Build history of the part. All positions in model axes, mm. A direction names the side the tool comes from. Round coordinates to 2 decimals unless told otherwise and drop trailing zeros. Write each loop counter-clockwise with the first axis right and the second up, starting at its lowest first coordinate (ties: lowest second). Pieces come first, ordered by that corner, then holes. Notation, with made-up numbers: M -38.75,66.25 L -1.75,66.25 A7 ccw -1.75,79.25 Z; hole C 47,-31.5 d10. An arc over 180 degrees is marked long. Write item = value, one per line. Start each with the question number.
Q1. Drop flat-ended pins along their axis: P1, Ø2.5, axis at x = -21.5, y = 1.5, coming from the +Z side; P2, Ø3.5, axis at y = 50.5, z = -25.11, coming from the -X side; P3, Ø5.5, axis at y = 1.5, z = 38.5, coming from the -X side; P4, Ø5.5, axis at x = -17.32, z = 10, coming from the -Y side. Give the stop position or say it passes through.
Q2. Band-saw the part on B-B on y = 8.5. State how many separate pieces and enclosed holes the cut face has, plus the area to 3 significant figures.
Q3. Tool access for faces 1 (the flat face through (-15, 10, 10)), 2 (the cylindrical face through (-16.27, 2.54, -42.79)), 3 (the flat face through (2, 10, -20)): list every direction of +Z, -Z, +X, -X, +Y, -Y with a clear straight run to the whole face (end or side of a thin tool).
Q4. Band-saw the part on A-A on z = 0. Write the cut outline in (x, y).
Q5. Pull direction Z, two halves, no side cores. Call faces 4 (the flat face through (19.5, 10, 10.1)), 5 (the flat face through (24, 23, -50)), 6 (the cylindrical face through (37.47, 48.46, 26.18)): released by +Z, released by -Z, zero draft, split by the parting line, or undercut.
Q6. Band-saw the part on C-C on x = 24.5. Write the cut outline in (y, z), plus the area to 3 significant figures.
Q7. Probe L1, parallel to Z at x = 0, y = 3.3; L2, parallel to Y at x = 38, z = 38; L3, parallel to Z at x = 36, y = 50. List the from-to ranges inside material, lowest first.
```python
from build123d import *

# Parameters (mm, degrees)
SKETCH_1_W          = 70
SKETCH_1_H          = 70
EXTRUDE_1_DEPTH     = 5
HOLE_WIZARD_1_D     = 3.5
HOLE_WIZARD_2_D     = 23
SKETCH_7_W          = 70
SKETCH_7_H          = 100
EXTRUDE_2_DEPTH     = 5
HOLE_WIZARD_4_D     = 4.6
HOLE_WIZARD_5_D     = 23
SKETCH_16_R         = 5
SKETCH_16_R_2       = 1.75
EXTRUDE_3_DEPTH     = 5
SKETCH_17_W         = 5
SKETCH_17_H         = 60
SKETCH_17_W_2       = 35
SKETCH_17_H_2       = 5
EXTRUDE_4_DEPTH     = 15
SKETCH_18_W         = 35
SKETCH_18_H         = 5
SKETCH_18_W_2       = 5
SKETCH_18_H_2       = 60
EXTRUDE_5_DEPTH     = 15
EXTRUDE_6_DEPTH     = 5
EXTRUDE_7_DEPTH     = 5
HOLE_WIZARD_6_D     = 3
HOLE_WIZARD_6_DEPTH = 5
FILLET_2_R          = 20
HOLE_WIZARD_7_D     = 9
CUT_EXTRUDE_1_DEPTH = 10
FILLET_3_R          = 2
FILLET_4_R          = 15
SKETCH_29_W         = 20
SKETCH_29_H         = 10
CUT_EXTRUDE_2_DEPTH = 10
FILLET_5_R          = 3
HOLE_WIZARD_8_D     = 3.3
CUT_EXTRUDE_3_REACH = 148.969


with BuildPart() as part:
    # 草图1 → 凸台-拉伸1 (new body)
    with BuildSketch(Plane(origin=(0, 0, 0), x_dir=(1, 0, 0), z_dir=(0, 1, 0))):
        Rectangle(SKETCH_1_W, SKETCH_1_H)
    extrude(amount=EXTRUDE_1_DEPTH)

    # 孔1 (through all)
    with Locations(Plane(origin=(0, 5, 0), x_dir=(1, 0, 0), z_dir=(0, 1, 0))):
        with Locations((0, 20), (-17.320508076, -10), (17.320508076, -10)):
            Hole(HOLE_WIZARD_1_D / 2)

    # 孔2 (through all)
    with Locations(Plane(origin=(0, 5, 0), x_dir=(1, 0, 0), z_dir=(0, 1, 0))):
        with Locations((0, 0)):
            Hole(HOLE_WIZARD_2_D / 2)

    # 草图7 → 凸台-拉伸2 (add)
    with BuildSketch(Plane(origin=(35, 0, 0), x_dir=(0, 0, -1), z_dir=(1, 0, 0))):
        with Locations((0, 50)):
            Rectangle(SKETCH_7_W, SKETCH_7_H)
    extrude(amount=EXTRUDE_2_DEPTH)

    # 孔4 (through all)
    with Locations(Plane(origin=(40, 0, 0), x_dir=(0, 0, -1), z_dir=(1, 0, 0))):
        with Locations((0, 94), (-25.11473671, 50.5), (25.11473671, 50.5)):
            Hole(HOLE_WIZARD_4_D / 2)

    # 孔5 (through all)
    with Locations(Plane(origin=(40, 0, 0), x_dir=(0, 0, -1), z_dir=(1, 0, 0))):
        with Locations((0, 65)):
            Hole(HOLE_WIZARD_5_D / 2)

    # 草图16 → 凸台-拉伸3 (add)
    # profile 1 of 3: a face of its own
    with BuildSketch(Plane(origin=(0, 5, 0), x_dir=(1, 0, 0), z_dir=(0, 1, 0))):
        with Locations(Location((0, 20, 0), (0, 0, 90))):
            Circle(SKETCH_16_R)
        with Locations(Location((0, 20, 0), (0, 0, 270))):
            Circle(SKETCH_16_R_2, mode=Mode.SUBTRACT)
    # profile 2 of 3: a face of its own
    with BuildSketch(Plane(origin=(0, 5, 0), x_dir=(1, 0, 0), z_dir=(0, 1, 0))):
        with Locations(Location((-17.320508076, -10, 0), (0, 0, 90))):
            Circle(SKETCH_16_R)
        with Locations(Location((-17.320508076, -10, 0), (0, 0, 270))):
            Circle(SKETCH_16_R_2, mode=Mode.SUBTRACT)
    # profile 3 of 3: a face of its own
    with BuildSketch(Plane(origin=(0, 5, 0), x_dir=(1, 0, 0), z_dir=(0, 1, 0))):
        with Locations(Location((17.320508076, -10, 0), (0, 0, 90))):
            Circle(SKETCH_16_R)
        with Locations(Location((17.320508076, -10, 0), (0, 0, 270))):
            Circle(SKETCH_16_R_2, mode=Mode.SUBTRACT)
    extrude(amount=EXTRUDE_3_DEPTH)

    # 草图17 → 凸台-拉伸4 (add)
    with BuildSketch(Plane(origin=(0, 0, -35), x_dir=(-1, 0, 0), z_dir=(0, 0, -1))):
        with Locations((-37.5, 70)):
            Rectangle(SKETCH_17_W, SKETCH_17_H)
        Polygon((-35, 35), (-40, 40), (-40, 0), (0, 0), (-5, 5), (-35, 5), align=None)
        Polygon((-35, 40), (-40, 40), (-35, 35), align=None)
        with Locations((17.5, 2.5)):
            Rectangle(SKETCH_17_W_2, SKETCH_17_H_2)
        Polygon((0, 5), (-5, 5), (0, 0), align=None)
    extrude(amount=EXTRUDE_4_DEPTH)

    # 草图18 → 凸台-拉伸5 (add)
    with BuildSketch(Plane.XY.offset(35)):
        with Locations((-17.5, 2.5)):
            Rectangle(SKETCH_18_W, SKETCH_18_H)
        Polygon((0, 0), (5, 5), (0, 5), align=None)
        Polygon((40, 0), (40, 40), (35, 35), (35, 5), (5, 5), (0, 0), align=None)
        Polygon((35, 35), (40, 40), (35, 40), align=None)
        with Locations((37.5, 70)):
            Rectangle(SKETCH_18_W_2, SKETCH_18_H_2)
    extrude(amount=EXTRUDE_5_DEPTH)

    # 草图19 → 凸台-拉伸6 (add)
    with BuildSketch(Plane(origin=(0, 0, -50), x_dir=(-1, 0, 0), z_dir=(0, 0, -1))):
        Polygon((15, 5), (-35, 64.58767963), (-35, 5), align=None)
    extrude(amount=-EXTRUDE_6_DEPTH)

    # 草图20 → 凸台-拉伸7 (add)
    with BuildSketch(Plane.XY.offset(50)):
        Polygon((-15, 5), (35, 64.58767963), (35, 5), align=None)
    extrude(amount=-EXTRUDE_7_DEPTH)

    # 孔6
    with Locations(Plane(origin=(40, 0, 0), x_dir=(0, 0, -1), z_dir=(1, 0, 0))):
        with Locations((-38.5, 57.5), (-38.5, 8.5), (19.5, 8.5)):
            Hole(HOLE_WIZARD_6_D / 2, depth=HOLE_WIZARD_6_DEPTH)

    # 圆角2
    # the kernel refuses this fillet: 20 mm, written as the material it takes off along each edge
    with BuildSketch(Plane(origin=(-15, 100, -50), x_dir=(0, -1, 0), z_dir=(1, 0, 0)), Plane(origin=(90, 100, 50), x_dir=(0, -1, 0), z_dir=(-1, 0, 0))) as fillet_2_piece_1:
        with BuildLine():
            CenterArc((FILLET_2_R, -FILLET_2_R), FILLET_2_R, 90, 90)
            Line((0, -FILLET_2_R), (0, 0))
            Line((0, 0), (FILLET_2_R, 0))
        make_face()
    extrude(amount=105, mode=Mode.SUBTRACT)

    # 孔7 (through all)
    with Locations(Plane.ZY.offset(-35)):
        with Locations((-16.670989023, 55.375)):
            Hole(HOLE_WIZARD_7_D / 2)

    # 草图28 → 切除-拉伸1 (cut)
    with BuildSketch(Plane(origin=(0, 5, 0), x_dir=(1, 0, 0), z_dir=(0, 1, 0))):
        Polygon((-15, 45.757359313), (-30.757359313, 30), (-15, 30), align=None)
        Polygon((-30.757359313, -30), (-15, -45.757359313), (-15, -30), align=None)
    extrude(amount=-CUT_EXTRUDE_1_DEPTH, mode=Mode.SUBTRACT)

    # 圆角3
    # the kernel refuses this fillet: 2 mm, written as the material it adds along each edge
    with BuildSketch(Plane(origin=(-30.757359313, 5, -30), x_dir=(0.7071067811865478, 0, -0.7071067811865471), z_dir=(0, -1, 0)), Plane(origin=(-15, 5, 45.757359313), x_dir=(-0.7071067811865471, 0, -0.7071067811865479), z_dir=(0, -1, 0))) as fillet_3_piece_1:
        with BuildLine():
            CenterArc((FILLET_3_R * 2.41421356237, FILLET_3_R), FILLET_3_R, 135, 135)
            Line((FILLET_3_R * 1.70710678119, FILLET_3_R * 1.70710678119), (0, 0))
            Line((0, 0), (FILLET_3_R * 2.41421356237, 0))
        make_face()
    extrude(amount=5)
    with BuildSketch(Plane(origin=(-15, 5, -45.757359313), x_dir=(-0.7071067811865478, 0, 0.7071067811865474), z_dir=(0, -1, 0)), Plane(origin=(-30.757359313, 5, 30), x_dir=(0.7071067811865476, 0, 0.7071067811865476), z_dir=(0, -1, 0))) as fillet_3_piece_2:
        with BuildLine():
            CenterArc((FILLET_3_R * 2.41421356237, -FILLET_3_R), FILLET_3_R, 90, 135)
            Line((FILLET_3_R * 1.70710678119, -FILLET_3_R * 1.70710678119), (0, 0))
            Line((0, 0), (FILLET_3_R * 2.41421356237, 0))
        make_face()
    extrude(amount=5)
    with BuildSketch(Plane(origin=(-15, 5, -30), x_dir=(-1, 0, 0), z_dir=(0, -1, 0)), Plane(origin=(-15, 5, 30), x_dir=(0, 0, 1), z_dir=(0, -1, 0))) as fillet_3_piece_3:
        with BuildLine():
            CenterArc((FILLET_3_R, FILLET_3_R), FILLET_3_R, 180, 90)
            Line((0, FILLET_3_R), (0, 0))
            Line((0, 0), (FILLET_3_R, 0))
        make_face()
    extrude(amount=5)

    # 圆角4
    fillet_4_edges = [part.edges().sort_by_distance(p)[0] for p in [
        (-35, 2.5, -50),
        (-35, 2.5, 50),
    ]]
    fillet(fillet_4_edges, radius=FILLET_4_R)

    # 草图29 → 切除-拉伸2 (cut)
    with BuildSketch(Plane(origin=(40, 0, 0), x_dir=(0, 0, -1), z_dir=(1, 0, 0))):
        with Locations((35, 10)):
            Rectangle(SKETCH_29_W, SKETCH_29_H)
    extrude(amount=-CUT_EXTRUDE_2_DEPTH, mode=Mode.SUBTRACT)

    # 圆角5
    fillet_5_edges = [part.edges().sort_by_distance(p)[0] for p in [
        (37.5, 15, -45),
        (37.5, 15, -25),
    ]]
    fillet(fillet_5_edges, radius=FILLET_5_R)

    # 孔8 (through all)
    with Locations(Plane(origin=(0, 5, 0), x_dir=(1, 0, 0), z_dir=(0, 1, 0))):
        with Locations((-31.363961031, 37.878679656), (-27.121320344, 42.121320344), (-22.878679656, 46.363961031)):
            Hole(HOLE_WIZARD_8_D / 2)

    # 草图34 → 切除-拉伸3 (cut, up to next)
    with BuildSketch(Plane.XY.offset(50), mode=Mode.PRIVATE) as cut_extrude_3_sk1:
        Polygon((35, 5), (35, 39.6960984), (5.886516629, 5), align=None)
    cut_extrude_3_tool1 = extrude(cut_extrude_3_sk1.sketch, amount=-CUT_EXTRUDE_3_REACH, mode=Mode.PRIVATE) & part.part
    add(cut_extrude_3_tool1.solids().sort_by_distance((25.295506, 16.565366, 50))[0], mode=Mode.SUBTRACT)


solid = part.part
```
Conclusion:
q1.P1 = 50
q1.P2 = through
q1.P3 = -34.98
q1.P4 = 0
q2.separate_pieces = 8
q2.enclosed_holes = 3
q2.area = 917 mm^2
q3.face_1 = +Z, -Z, -X, +Y
q3.face_2 = +Y, -Y
q3.face_3 = -X, +Y
q4.outline = M -35,0 L -11.5,0 L -11.5,5 L -35,5 Z; M 11.5,0 L 40,0 L 40,53.5 L 35,53.5 L 35,5 L 11.5,5 Z; M 35,76.5 L 40,76.5 L 40,91.7 L 35,91.7 Z; M 35,96.3 L 40,96.3 L 40,100 L 35,100 Z
q5.face_4 = zero draft
q5.face_5 = released by -Z
q5.face_6 = undercut
q6.outline = M 0,-50 L 52.07,-50 L 52.07,-45 L 5,-45 L 5,50 L 0,50 Z; M 27.18,45 L 52.07,45 L 52.07,50 L 27.18,50 Z
q6.area = 860 mm^2
q7.L1 = -50 to -21.75, -18.25 to -11.5, 11.5 to 50
q7.L2 = 0 to 7.09, 9.91 to 56.09, 58.91 to 98.33
q7.L3 = -50 to -27.36, -22.87 to 22.87, 27.36 to 50
